Source: CAD feature listing. Evaluate the final solid. Frame: model axes, mm. Face numbers are marked on the shaded views. Give positions to 0.01 mm unless a question says otherwise; leave off trailing zeros. Loops run counter-clockwise (first coordinate to the right, second up) from the corner with the lowest first, then second, coordinate; pieces in that order, holes last.
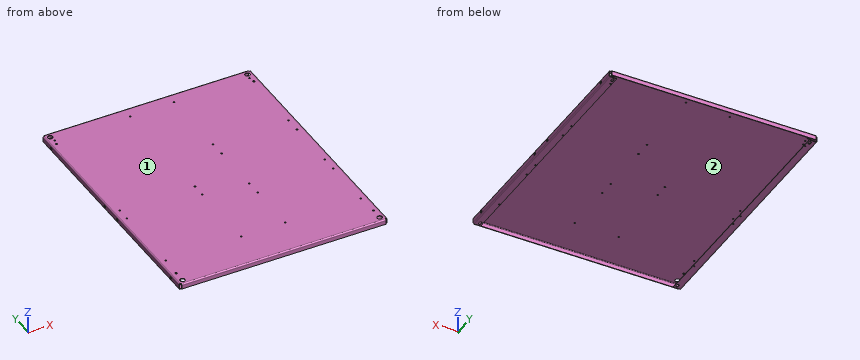
from build123d import *

# Parameters (mm, degrees)
ESQUISSE1_W                                   = 896
ESQUISSE1_H                                   = 1080.9248
BOSS_EXTRU_1_DEPTH                            = 27
ENL_V_MAT_EXTRU_1_DEPTH                       = 1081.9248
ESQUISSE3_W                                   = 879.9248
ESQUISSE3_H                                   = 2.5
BOSS_EXTRU_2_DEPTH                            = 8.0376
ESQUISSE4_W                                   = 879.9248
ESQUISSE4_H                                   = 2.5
BOSS_EXTRU_3_DEPTH                            = 19.5
ESQUISSE5_W                                   = 879.9248
ESQUISSE5_H                                   = 2.5
BOSS_EXTRU_4_DEPTH                            = 8.0376
ESQUISSE6_W                                   = 879.9248
ESQUISSE6_H                                   = 2.5
BOSS_EXTRU_5_DEPTH                            = 19.5
ENL_V_MAT_EXTRU_2_REACH                       = 29
ENL_V_MAT_EXTRU_3_DEPTH                       = 3.5
ENL_V_MAT_EXTRU_4_DEPTH                       = 3.5
ENL_V_MAT_EXTRU_5_DEPTH                       = 3.5
ENL_V_MAT_EXTRU_6_DEPTH                       = 3.5
ENL_V_MAT_EXTRU_7_DEPTH                       = 3.5
ENL_V_MAT_EXTRU_8_DEPTH                       = 3.5
ENL_V_MAT_EXTRU_9_REACH                       = 898
ENL_V_MAT_EXTRU_10_REACH                      = 898
ENL_V_MAT_EXTRU_11_REACH                      = 898
ENL_V_MAT_EXTRU_12_REACH                      = 898
ENL_V_MAT_EXTRU_13_REACH                      = 29
DIAM_TRE_DU_PER_AGE_9_0_9_1_D                 = 9
DIAM_TRE_DU_PER_AGE_9_0_9_1_DEPTH             = 2.5
DIAM_TRE_DU_PER_AGE_22_0_22_1_D               = 22
DIAM_TRE_DU_PER_AGE_22_0_22_1_DEPTH           = 2.5
CONG_1_R                                      = 3
CONG_2_R                                      = 5.5
TROU_POUR_TARAUDAGE_POUR_TROU_TARAUD_M8_D     = 6.8
TROU_POUR_TARAUDAGE_POUR_TROU_TARAUD_M8_DEPTH = 40
TROU_POUR_TARAUDAGE_POUR_TROU_TARAUD_M8_TIP   = 2.042926105
TROU_POUR_TARAUDAGE_POUR_TROU_TARAUD_2_D      = 6.8
TROU_POUR_TARAUDAGE_POUR_TROU_TARAUD_2_DEPTH  = 40
TROU_POUR_TARAUDAGE_POUR_TROU_TARAUD_2_TIP    = 2.042926105


with BuildPart() as part:
    # Esquisse1 → Boss.-Extru.1 (new body)
    with BuildSketch(Plane.XY):
        Rectangle(ESQUISSE1_W, ESQUISSE1_H)
    extrude(amount=-BOSS_EXTRU_1_DEPTH)

    # Esquisse2 → Enlèv. mat.-Extru.1 (cut, through all)
    with BuildSketch(Plane(origin=(0, 540.4624, 0), x_dir=(-1, 0, 0), z_dir=(0, 1, 0))):
        Polygon((415, -27), (415, -24.5), (445.5, -24.5), (445.5, -2.5), (-445.5, -2.5), (-445.5, -24.5), (-415, -24.5), (-415, -27), align=None)
    extrude(amount=-ENL_V_MAT_EXTRU_1_DEPTH, mode=Mode.SUBTRACT)

    # Esquisse3 → Boss.-Extru.2 (add)
    with BuildSketch(Plane.XZ.offset(540.4624)):
        with Locations((0, -1.25)):
            Rectangle(ESQUISSE3_W, ESQUISSE3_H)
    extrude(amount=BOSS_EXTRU_2_DEPTH)

    # Esquisse4 → Boss.-Extru.3 (add)
    with BuildSketch(Plane(origin=(0, 0, -2.5), x_dir=(-1, 0, 0), z_dir=(0, 0, -1))):
        with Locations((0, -547.25)):
            Rectangle(ESQUISSE4_W, ESQUISSE4_H)
    extrude(amount=BOSS_EXTRU_3_DEPTH)

    # Esquisse5 → Boss.-Extru.4 (add)
    with BuildSketch(Plane(origin=(0, 540.4624, 0), x_dir=(-1, 0, 0), z_dir=(0, 1, 0))):
        with Locations((0, -1.25)):
            Rectangle(ESQUISSE5_W, ESQUISSE5_H)
    extrude(amount=BOSS_EXTRU_4_DEPTH)

    # Esquisse6 → Boss.-Extru.5 (add)
    with BuildSketch(Plane(origin=(0, 0, -2.5), x_dir=(-1, 0, 0), z_dir=(0, 0, -1))):
        with Locations((0, 547.25)):
            Rectangle(ESQUISSE6_W, ESQUISSE6_H)
    extrude(amount=BOSS_EXTRU_5_DEPTH)

    # Esquisse7 → Enlèv. mat.-Extru.2 (cut, up to next)
    with BuildSketch(Plane(origin=(0, 0, -27), x_dir=(-1, 0, 0), z_dir=(0, 0, -1)), mode=Mode.PRIVATE) as enl_v_mat_extru_2_sk1:
        with BuildLine():
            Line((-430, -521), (-430, -529))
            ThreePointArc((-430, -529), (-425, -534), (-420, -529))
            Line((-420, -529), (-420, -521))
            ThreePointArc((-420, -521), (-425, -516), (-430, -521))
        make_face()
    enl_v_mat_extru_2_tool1 = extrude(enl_v_mat_extru_2_sk1.sketch, amount=-ENL_V_MAT_EXTRU_2_REACH, mode=Mode.PRIVATE) & part.part
    add(enl_v_mat_extru_2_tool1.solids().sort_by_distance((425, -525, -27))[0], mode=Mode.SUBTRACT)

    # Esquisse8 → Enlèv. mat.-Extru.3 (cut, through all)
    with BuildSketch(Plane.ZY.offset(-445.5)):
        with BuildLine():
            Line((-9, -52), (-9, -48))
            ThreePointArc((-9, -48), (-13.5, -43.5), (-18, -48))
            Line((-18, -48), (-18, -52))
            ThreePointArc((-18, -52), (-13.5, -56.5), (-9, -52))
        make_face()
    extrude(amount=-ENL_V_MAT_EXTRU_3_DEPTH, mode=Mode.SUBTRACT)

    # Esquisse9 → Enlèv. mat.-Extru.4 (cut, through all)
    with BuildSketch(Plane.ZY.offset(-445.5)):
        with BuildLine():
            Line((-11.5, -470.5), (-15.5, -470.5))
            ThreePointArc((-15.5, -470.5), (-20, -475), (-15.5, -479.5))
            Line((-15.5, -479.5), (-11.5, -479.5))
            ThreePointArc((-11.5, -479.5), (-7, -475), (-11.5, -470.5))
        make_face()
    extrude(amount=-ENL_V_MAT_EXTRU_4_DEPTH, mode=Mode.SUBTRACT)

    # Esquisse10 → Enlèv. mat.-Extru.5 (cut, through all)
    with BuildSketch(Plane.ZY.offset(-445.5)):
        with BuildLine():
            Line((-11.5, 479.5), (-15.5, 479.5))
            ThreePointArc((-15.5, 479.5), (-20, 475), (-15.5, 470.5))
            Line((-15.5, 470.5), (-11.5, 470.5))
            ThreePointArc((-11.5, 470.5), (-7, 475), (-11.5, 479.5))
        make_face()
    extrude(amount=-ENL_V_MAT_EXTRU_5_DEPTH, mode=Mode.SUBTRACT)

    # Esquisse11 → Enlèv. mat.-Extru.6 (cut, through all)
    with BuildSketch(Plane.ZY.offset(-445.5)):
        with BuildLine():
            Line((-11.5, 54.5), (-15.5, 54.5))
            ThreePointArc((-15.5, 54.5), (-20, 50), (-15.5, 45.5))
            Line((-15.5, 45.5), (-11.5, 45.5))
            ThreePointArc((-11.5, 45.5), (-7, 50), (-11.5, 54.5))
        make_face()
    extrude(amount=-ENL_V_MAT_EXTRU_6_DEPTH, mode=Mode.SUBTRACT)

    # Esquisse12 → Enlèv. mat.-Extru.7 (cut, through all)
    with BuildSketch(Plane.XY.offset(-24.5)):
        with BuildLine():
            Line((430, 521), (430, 529))
            ThreePointArc((430, 529), (425, 534), (420, 529))
            Line((420, 529), (420, 521))
            ThreePointArc((420, 521), (425, 516), (430, 521))
        make_face()
    extrude(amount=-ENL_V_MAT_EXTRU_7_DEPTH, mode=Mode.SUBTRACT)

    # Esquisse13 → Enlèv. mat.-Extru.8 (cut, through all)
    with BuildSketch(Plane.XY.offset(-24.5)):
        with BuildLine():
            Line((-430, -521), (-430, -529))
            ThreePointArc((-430, -529), (-425, -534), (-420, -529))
            Line((-420, -529), (-420, -521))
            ThreePointArc((-420, -521), (-425, -516), (-430, -521))
        make_face()
    extrude(amount=-ENL_V_MAT_EXTRU_8_DEPTH, mode=Mode.SUBTRACT)

    # Esquisse14 → Enlèv. mat.-Extru.9 (cut, up to next)
    with BuildSketch(Plane.ZY.offset(448), mode=Mode.PRIVATE) as enl_v_mat_extru_9_sk1:
        with BuildLine():
            Line((-11.5, -45.5), (-15.5, -45.5))
            ThreePointArc((-15.5, -45.5), (-20, -50), (-15.5, -54.5))
            Line((-15.5, -54.5), (-11.5, -54.5))
            ThreePointArc((-11.5, -54.5), (-7, -50), (-11.5, -45.5))
        make_face()
    enl_v_mat_extru_9_tool1 = extrude(enl_v_mat_extru_9_sk1.sketch, amount=-ENL_V_MAT_EXTRU_9_REACH, mode=Mode.PRIVATE) & part.part
    add(enl_v_mat_extru_9_tool1.solids().sort_by_distance((-448, -50, -13.5))[0], mode=Mode.SUBTRACT)

    # Esquisse15 → Enlèv. mat.-Extru.10 (cut, up to next)
    with BuildSketch(Plane.ZY.offset(448), mode=Mode.PRIVATE) as enl_v_mat_extru_10_sk1:
        with BuildLine():
            Line((-9, -477), (-9, -473))
            ThreePointArc((-9, -473), (-13.5, -468.5), (-18, -473))
            Line((-18, -473), (-18, -477))
            ThreePointArc((-18, -477), (-13.5, -481.5), (-9, -477))
        make_face()
    enl_v_mat_extru_10_tool1 = extrude(enl_v_mat_extru_10_sk1.sketch, amount=-ENL_V_MAT_EXTRU_10_REACH, mode=Mode.PRIVATE) & part.part
    add(enl_v_mat_extru_10_tool1.solids().sort_by_distance((-448, -475, -13.5))[0], mode=Mode.SUBTRACT)

    # Esquisse16 → Enlèv. mat.-Extru.11 (cut, up to next)
    with BuildSketch(Plane.ZY.offset(448), mode=Mode.PRIVATE) as enl_v_mat_extru_11_sk1:
        with BuildLine():
            Line((-9, 473), (-9, 477))
            ThreePointArc((-9, 477), (-13.5, 481.5), (-18, 477))
            Line((-18, 477), (-18, 473))
            ThreePointArc((-18, 473), (-13.5, 468.5), (-9, 473))
        make_face()
    enl_v_mat_extru_11_tool1 = extrude(enl_v_mat_extru_11_sk1.sketch, amount=-ENL_V_MAT_EXTRU_11_REACH, mode=Mode.PRIVATE) & part.part
    add(enl_v_mat_extru_11_tool1.solids().sort_by_distance((-448, 475, -13.5))[0], mode=Mode.SUBTRACT)

    # Esquisse17 → Enlèv. mat.-Extru.12 (cut, up to next)
    with BuildSketch(Plane.ZY.offset(448), mode=Mode.PRIVATE) as enl_v_mat_extru_12_sk1:
        with BuildLine():
            Line((-9, 48), (-9, 52))
            ThreePointArc((-9, 52), (-13.5, 56.5), (-18, 52))
            Line((-18, 52), (-18, 48))
            ThreePointArc((-18, 48), (-13.5, 43.5), (-9, 48))
        make_face()
    enl_v_mat_extru_12_tool1 = extrude(enl_v_mat_extru_12_sk1.sketch, amount=-ENL_V_MAT_EXTRU_12_REACH, mode=Mode.PRIVATE) & part.part
    add(enl_v_mat_extru_12_tool1.solids().sort_by_distance((-448, 50, -13.5))[0], mode=Mode.SUBTRACT)

    # Esquisse18 → Enlèv. mat.-Extru.13 (cut, up to next)
    with BuildSketch(Plane(origin=(0, 0, -27), x_dir=(-1, 0, 0), z_dir=(0, 0, -1)), mode=Mode.PRIVATE) as enl_v_mat_extru_13_sk1:
        with BuildLine():
            Line((430, 521), (430, 529))
            ThreePointArc((430, 529), (425, 534), (420, 529))
            Line((420, 529), (420, 521))
            ThreePointArc((420, 521), (425, 516), (430, 521))
        make_face()
    enl_v_mat_extru_13_tool1 = extrude(enl_v_mat_extru_13_sk1.sketch, amount=-ENL_V_MAT_EXTRU_13_REACH, mode=Mode.PRIVATE) & part.part
    add(enl_v_mat_extru_13_tool1.solids().sort_by_distance((-425, 525, -27))[0], mode=Mode.SUBTRACT)

    # Diamètre du perçage Ø9.0 (9)1
    with Locations(Plane(origin=(0, 0, -2.5), x_dir=(-1, 0, 0), z_dir=(0, 0, -1))):
        with Locations((425, -475), (425, 475), (-425, -475), (-425, 475)):
            Hole(DIAM_TRE_DU_PER_AGE_9_0_9_1_D / 2, depth=DIAM_TRE_DU_PER_AGE_9_0_9_1_DEPTH)

    # Diamètre du perçage Ø22.0 (22)1
    with Locations(Plane(origin=(0, 0, -2.5), x_dir=(-1, 0, 0), z_dir=(0, 0, -1))):
        with Locations((425, -525), (425, 525), (-425, -525), (-425, 525)):
            Hole(DIAM_TRE_DU_PER_AGE_22_0_22_1_D / 2, depth=DIAM_TRE_DU_PER_AGE_22_0_22_1_DEPTH)

    # Congé1
    cong_1_edges = [part.edges().sort_by_distance(p)[0] for p in [
        (445.5, 0, -24.5),
        (445.5, 0, -2.5),
        (-445.5, 0, -2.5),
        (-445.5, 0, -24.5),
        (0, -546, -2.5),
        (0, 546, -2.5),
    ]]
    fillet(cong_1_edges, radius=CONG_1_R)

    # Congé2
    cong_2_edges = [part.edges().sort_by_distance(p)[0] for p in [
        (448, 0, -27),
        (448, 0, 0),
        (0, -548.5, 0),
        (-448, 0, 0),
        (-448, 0, -27),
        (0, 548.5, 0),
    ]]
    fillet(cong_2_edges, radius=CONG_2_R)

    # Trou pour taraudage pour trou taraud_ M8
    with Locations(Plane.XY):
        with Locations((-420, 498.5)):
            Hole(TROU_POUR_TARAUDAGE_POUR_TROU_TARAUD_M8_D / 2, depth=TROU_POUR_TARAUDAGE_POUR_TROU_TARAUD_M8_DEPTH)
            with Locations((0, 0, -(TROU_POUR_TARAUDAGE_POUR_TROU_TARAUD_M8_DEPTH + TROU_POUR_TARAUDAGE_POUR_TROU_TARAUD_M8_TIP / 2))):  # 118° drill point
                Cone(0, TROU_POUR_TARAUDAGE_POUR_TROU_TARAUD_M8_D / 2, TROU_POUR_TARAUDAGE_POUR_TROU_TARAUD_M8_TIP, mode=Mode.SUBTRACT)

    # Trou pour taraudage pour trou taraud 2
    with Locations(Plane.XY):
        with Locations((-95, 498.5), (95, 501), (420, 501), (420, 191), (420, 123.5), (95, 191), (95, 123.5), (95, -96.5), (95, -164), (420, -96.5), (420, -164), (420, -384), (95, -384), (-95, -384), (-420, -384), (-420, -74), (-420, -16.5), (-95, -16.5), (-95, -74)):
            Hole(TROU_POUR_TARAUDAGE_POUR_TROU_TARAUD_2_D / 2, depth=TROU_POUR_TARAUDAGE_POUR_TROU_TARAUD_2_DEPTH)
            with Locations((0, 0, -(TROU_POUR_TARAUDAGE_POUR_TROU_TARAUD_2_DEPTH + TROU_POUR_TARAUDAGE_POUR_TROU_TARAUD_2_TIP / 2))):  # 118° drill point
                Cone(0, TROU_POUR_TARAUDAGE_POUR_TROU_TARAUD_2_D / 2, TROU_POUR_TARAUDAGE_POUR_TROU_TARAUD_2_TIP, mode=Mode.SUBTRACT)


solid = part.part
1) Cut plane B-B (y = -305.5). Return loops of the section in (x, z), and give its area (3 significant figures).
Checks:
outline: (-448, -21.5) arc R5.5 ccw to (-442.5, -27) - (-415, -27) - (-415, -24.5) - (-442.5, -24.5) arc R3 cw to (-445.5, -21.5) - (-445.5, -5.5) arc R3 cw to (-442.5, -2.5) - (442.5, -2.5) arc R3 cw to (445.5, -5.5) - (445.5, -21.5) arc R3 cw to (442.5, -24.5) - (415, -24.5) - (415, -27) - (442.5, -27) arc R5.5 ccw to (448, -21.5) - (448, -5.5) arc R5.5 ccw to (442.5, 0) - (-442.5, 0) arc R5.5 ccw to (-448, -5.5) - close
area: 2,500 mm2
2) Contact query for flat-ended pins moving along their axis: P1, Ø11, axis at x = 95, y = -384, coming from the -Z side; P2, Ø2, axis at x = 446.5, z = -12.5, coming from the -Y side; P3, Ø0.8, axis at y = 526, z = -26, coming from the -X side. Output: stop coordinate, or through.
Checks:
P1: stops at z = -2.5
P2: stops at y = -540.46
P3: stops at x = -446.17
3) Ray query, probe 1 along X at (y, z) = (191, -1); probe 2 along Y at (x, z) = (-175.5, -8.75); probe 3 along X at (y, z) = (386, -16.75). Return the intervals inside material, ascending.
Checks:
probe 1: x = -445.66 to 91.6, 98.4 to 416.6, 423.4 to 445.66
probe 2: y = -548.5 to -546, 546 to 548.5
probe 3: x = -448 to -445.5, 445.5 to 448
4) Pull-direction query (Y, two-part tool) for the marked faces 1 and 2; classes: released by +Y, released by -Y, zero draft, split by the parting line, or undercut.
Checks:
face 1: zero draft
face 2: undercut
5) Cut plane A-A (x = -299). Return loops of the section in (y, z), and give its area (3 significant figures).
Checks:
outline: (-548.5, -22) - (-546, -22) - (-546, -5.5) arc R3 cw to (-543, -2.5) - (543, -2.5) arc R3 cw to (546, -5.5) - (546, -22) - (548.5, -22) - (548.5, -5.5) arc R5.5 ccw to (543, 0) - (-543, 0) arc R5.5 ccw to (-548.5, -5.5) - close
area: 2,830 mm2
